from build123d import *

# Parameters (mm, degrees)
SKETCH_1_W      = 5.4
SKETCH_1_H      = 5.4
EXTRUDE_1_DEPTH = 2
SKETCH_2_R      = 12.313072817
SKETCH_2_R_2    = 10.813072817
EXTRUDE_2_DEPTH = 3
SKETCH_3_R      = 5.5
SKETCH_3_W      = 5.4
SKETCH_3_H      = 5.4
EXTRUDE_3_DEPTH = 6.2


with BuildPart() as part:
    # 스케치1 → 보스-돌출1 (new body)
    with BuildSketch(Plane(origin=(0, 0, 0), x_dir=(0, 1, 0), z_dir=(0, 0, 1))):
        with BuildLine():
            ThreePointArc((0.981635498, 12.273880965), (0, 12.75), (-0.981635498, 12.273880965))
            ThreePointArc((-0.981635498, 12.273880965), (-7.237442612, 9.961485162), (-11.369812421, 4.726428642))
            ThreePointArc((-11.369812421, 4.726428642), (-12.125970583, 3.939966678), (-11.976496524, 2.859246968))
            ThreePointArc((-11.976496524, 2.859246968), (-11.710428139, -3.804948754), (-8.00856602, -9.352787419))
            ThreePointArc((-8.00856602, -9.352787419), (-7.494261967, -10.314966678), (-6.42024642, -10.506769157))
            ThreePointArc((-6.42024642, -10.506769157), (0, -12.313072817), (6.42024642, -10.506769157))
            ThreePointArc((6.42024642, -10.506769157), (7.494261967, -10.314966678), (8.00856602, -9.352787419))
            ThreePointArc((8.00856602, -9.352787419), (11.710428139, -3.804948754), (11.976496524, 2.859246968))
            ThreePointArc((11.976496524, 2.859246968), (12.125970583, 3.939966678), (11.369812421, 4.726428642))
            ThreePointArc((11.369812421, 4.726428642), (7.237442612, 9.961485162), (0.981635498, 12.273880965))
        make_face()
        with BuildLine():
            ThreePointArc((5.733695154, 9.167730561), (0, 10.813072817), (-5.733695154, 9.167730561))
            Line((-5.733695154, 9.167730561), (-2.811327739, 5.145436885))
            ThreePointArc((-2.811327739, 5.145436885), (0, 5.863368008), (2.811327739, 5.145436885))
            Line((2.811327739, 5.145436885), (5.733695154, 9.167730561))
        make_face(mode=Mode.SUBTRACT)
        with BuildLine():
            ThreePointArc((10.490839132, -2.620083596), (10.283843364, 3.341423262), (6.947220646, 8.286052682))
            Line((6.947220646, 8.286052682), (4.024853231, 4.263759007))
            ThreePointArc((4.024853231, 4.263759007), (5.576394352, 1.811880359), (5.762349327, -1.083704125))
            Line((5.762349327, -1.083704125), (10.490839132, -2.620083596))
        make_face(mode=Mode.SUBTRACT)
        Rectangle(SKETCH_1_W, SKETCH_1_H, mode=Mode.SUBTRACT)
        with BuildLine():
            Line((-5.298823836, -2.510288899), (-10.027313641, -4.04666837))
            ThreePointArc((-10.027313641, -4.04666837), (-6.355764734, -8.747959671), (-0.75, -10.787031276))
            Line((-0.75, -10.787031276), (-0.75, -5.815202868))
            ThreePointArc((-0.75, -5.815202868), (-3.446401244, -4.743564363), (-5.298823836, -2.510288899))
        make_face(mode=Mode.SUBTRACT)
        with BuildLine():
            Line((-4.024853231, 4.263759007), (-6.947220646, 8.286052682))
            ThreePointArc((-6.947220646, 8.286052682), (-10.283843364, 3.341423262), (-10.490839132, -2.620083596))
            Line((-10.490839132, -2.620083596), (-5.762349327, -1.083704125))
            ThreePointArc((-5.762349327, -1.083704125), (-5.576394352, 1.811880359), (-4.024853231, 4.263759007))
        make_face(mode=Mode.SUBTRACT)
        with BuildLine():
            Line((0.75, -5.815202868), (0.75, -10.787031276))
            ThreePointArc((0.75, -10.787031276), (6.355764734, -8.747959671), (10.027313641, -4.04666837))
            Line((10.027313641, -4.04666837), (5.298823836, -2.510288899))
            ThreePointArc((5.298823836, -2.510288899), (3.446401244, -4.743564363), (0.75, -5.815202868))
        make_face(mode=Mode.SUBTRACT)
    extrude(amount=EXTRUDE_1_DEPTH)

    # 스케치2 → 보스-돌출2 (add)
    with BuildSketch(Plane.XY.offset(2)):
        Circle(SKETCH_2_R)
        Circle(SKETCH_2_R_2, mode=Mode.SUBTRACT)
    extrude(amount=EXTRUDE_2_DEPTH)

    # 스케치3 → 보스-돌출3 (add)
    with BuildSketch(Plane.XY.offset(2)):
        Circle(SKETCH_3_R)
        Rectangle(SKETCH_3_W, SKETCH_3_H, mode=Mode.SUBTRACT)
    extrude(amount=EXTRUDE_3_DEPTH)


solid = part.part
Can you work these out from the model? Positions are in its coordinate system, mm. A direction names the side the tool comes from. Give positions to 0.01 mm unless a question says otherwise; leave off trailing zeros. Order: outer loops, then holes, each group sorted by start corner. A loop starts at its lowest first (then second) coordinate and runs counter-clockwise, first axis right, second up. Notation, with made-up numbers: M 5,-3 L 62,-3 A38 ccw 62,36 Z; hole C -13.5,-24.5 d3. An arc over 180 degrees is marked long. Use a Markdown table: item, result. Add a question column.
Item 1: If I drill on L1, parallel to Y at x = 0, z = 3.65; L2, parallel to Y at x = -2.75, z = 1; L3, parallel to Y at x = 7, z = 1.5, over which ranges is the centre line in solid material (lowest first)? Write a range as [from, to].
Item 2: Suppose I cut it at A-A (z = 3.25). List the corners of the cut face in (x, y) for me, then the cut area to 3 significant figures.
Item 3: Suppose I cut it at B-B (x = 0). List the corners of the cut face in (y, z) for me.
Item 4: For faces 1 (the flat face through (0, -11, 5)), 2 (the flat face through (0, -3, 0)), 3 (the cylindrical face through (4.72, 3.48, 0.99)), which set-ups out of +Z, -Z, +X, -X, +Y, -Y let a thin tool reach every point of the face, with its end or its side?
Item 5: Suppose I cut it at D-D (z = 7). List the corners of the cut face in (x, y) for me, then the cut area to 3 significant figures.
Item 6: Suppose I cut it at C-C (x = 6.25). List the corners of the cut face in (y, z) for me.
Item 7: We'd pull the mould along X, two halves only. Please class faces 4 (the cylindrical face through (-1.19, -5.37, 5.06)), 5 (the flat face through (4, 0, 8.2)), 6 (the cylindrical face through (10.324, 7.481, 0.986)), 7 (the cylindrical face through (-5.863, -0.041, 0.986)): +X half, -X half, draft (parallel to the pull), parting line (faces both ways), or undercut.
Item 8: Will these pins go through, and if not, where does the flat tip stop? pin 1 (0.9 mm diameter, centred on x = -4, y = 11.5, fed in from +Z); pin 2 (2.5 mm diameter, centred on x = -0.5, z = 3, fed in from -Y); pin 3 (3 mm diameter, centred on x = -8, z = 3, fed in from -Y); pin 4 (1 mm diameter, centred on x = 8.5, z = 1, fed in from +Y).
Answer sheet:
| question | item | result |
|---|---|---|
| 1 | L1 | y = [-12.31, -10.81], [-5.5, -2.7], [2.7, 5.5], [10.81, 12.31] |
| 1 | L2 | y = [-12, -10.46], [-5.18, 5.18], [10.46, 12] |
| 1 | L3 | y = [-10.13, -8.24], [-0.75, 0.75], [8.24, 10.13] |
| 2 | outline | C 0,0 d24.63; C 0,0 d11; hole C 0,0 d21.63; hole M -2.7,-2.7 L 2.7,-2.7 L 2.7,2.7 L -2.7,2.7 Z |
| 2 | area | 175 mm² |
| 3 | outline | M -12.31,0 L -10.81,0 L -10.81,5 L -12.31,5 Z; M -5.86,0 L -2.7,0 L -2.7,8.2 L -5.5,8.2 L -5.5,2 L -5.86,2 Z; M 2.7,0 L 5.86,0 L 5.86,2 L 5.5,2 L 5.5,8.2 L 2.7,8.2 Z; M 10.81,0 L 12.31,0 L 12.31,5 L 10.81,5 Z |
| 4 | face 1 | +Z |
| 4 | face 2 | -Z, +X, -X, +Y, -Y |
| 4 | face 3 | +Z, -Z |
| 5 | outline | C 0,0 d11; hole M -2.7,-2.7 L 2.7,-2.7 L 2.7,2.7 L -2.7,2.7 Z |
| 5 | area | 65.9 mm² |
| 6 | outline | M -10.61,0 L -8.82,0 L -8.82,5 L -10.61,5 Z; M -0.75,0 L 0.75,0 L 0.75,2 L -0.75,2 Z; M 8.82,0 L 10.61,0 L 10.61,5 L 8.82,5 Z |
| 7 | face 4 | undercut |
| 7 | face 5 | draft |
| 7 | face 6 | +X half |
| 7 | face 7 | undercut |
| 8 | pin 1 | stops at z = 5 |
| 8 | pin 2 | stops at y = -12.31 |
| 8 | pin 3 | stops at y = -10.46 |
| 8 | pin 4 | stops at y = 9.36 |
